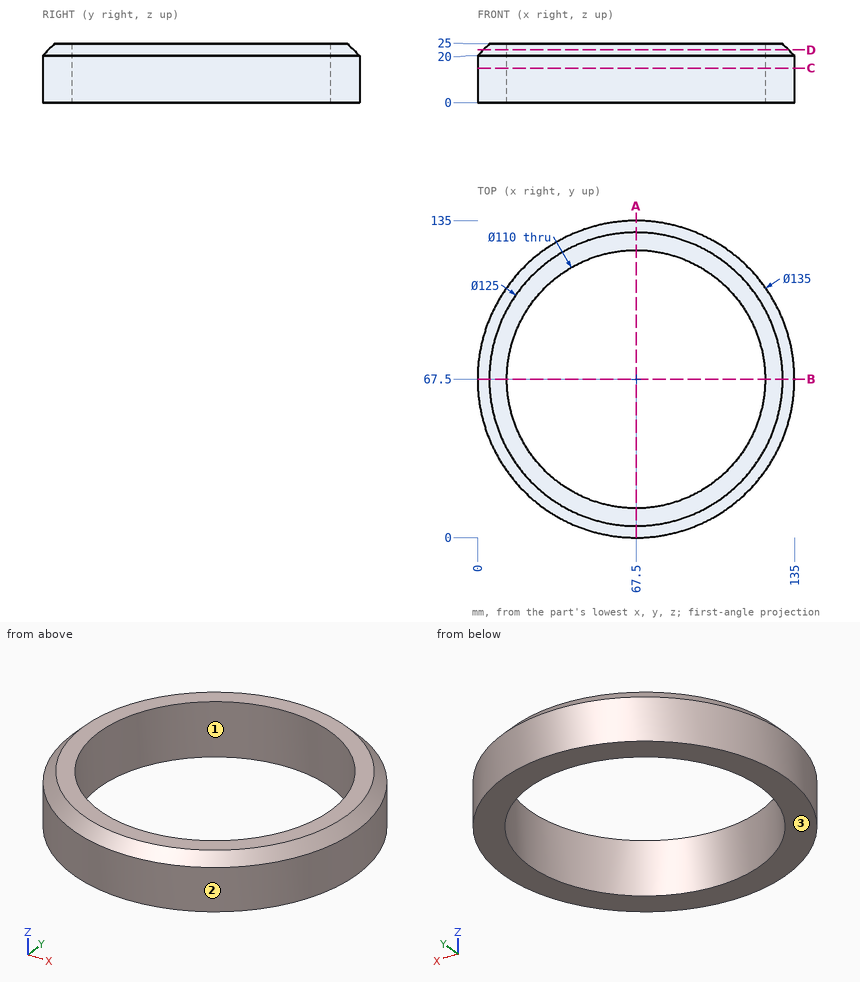
Here's the drawing with two shaded views (mm, measured from the low corner). I have some questions. Coordinates: 2 decimals unless noted, no trailing zeros. Write each loop counter-clockwise with the first axis right and the second up, starting at its lowest first coordinate (ties: lowest second). Pieces come first, ordered by that corner, then holes. Notation, with made-up numbers: M 19.25,72 L 49.25,72 A19 ccw 49.25,89 Z; hole C 71,45.5 d6. An arc over 180 degrees is marked long. Answer as CSV lines item,"result". Start each with the question number.
1) I want a section at D-D, the plane z = 22.5. Please give me the cut outline in (x, y).
2) We'd pull the mould along X, two halves only. Please class the marked faces 1, 2 and 3: +X half, -X half, draft (parallel to the pull), parting line (faces both ways), or undercut.
3) Please list where these lines run through material, in increasing order: line 1 (Y direction, x = 67.5, z = 8.5); line 2 (X direction, y = 32, z = 5); line 3 (Y direction, x = 48, z = 19). Write a range as from..to.
4) For P1, Ø8, axis at x = 42, z = 18.5, coming from the -Y side; P2, Ø12, axis at x = 42.5, z = 21.5, coming from the -Y side; P3, Ø10, axis at x = 73, z = 4, coming from the +Y side, each with a flat end and sliding along its axis, tell me the tip position at first contact or that it passes through.
5) I want a section at A-A, the plane x = 67.5. Please give me the cut outline in (y, z), and give its area (3 significant figures).
6) I want a section at C-C, the plane z = 14.75. Please give me the cut outline in (x, y).
Data:
1,outline,"C 67.5,67.5 d130; hole C 67.5,67.5 d110"
2,face 1,"undercut"
2,face 2,"parting line"
2,face 3,"draft"
3,line 1,"y = 0..12.5, 122.5..135"
3,line 2,"x = 10.09..25.49, 109.51..124.91"
3,line 3,"y = 2.88..16.07, 118.93..132.12"
4,P1,"stops at y = 3.52"
4,P2,"stops at y = 2.79"
4,P3,"stops at y = 135"
5,outline,"M 0,0 L 12.5,0 L 12.5,25 L 5,25 L 0,20 Z; M 122.5,0 L 135,0 L 135,20 L 130,25 L 122.5,25 Z"
5,area,"600 mm^2"
6,outline,"C 67.5,67.5 d135; hole C 67.5,67.5 d110"
